from build123d import *

# Parameters (mm, degrees)
SKETCH1_R           = 10
SKETCH1_R_2         = 5
BOSS_EXTRUDE1_DEPTH = 3
SKETCH1_3_R         = 5
BOSS_EXTRUDE2_DEPTH = 27
CHAMFER1_SIZE       = 1
FILLET1_R           = 1


with BuildPart() as part:
    # Sketch1 → Boss-Extrude1 (new body)
    # profile 1 of 2: a face of its own
    with BuildSketch(Plane.XY):
        Circle(SKETCH1_R)
        Circle(SKETCH1_R_2, mode=Mode.SUBTRACT)
    # profile 2 of 2: a face of its own
    with BuildSketch(Plane.XY):
        Circle(SKETCH1_R_2)
    extrude(amount=BOSS_EXTRUDE1_DEPTH)

    # Sketch1_3 → Boss-Extrude2 (add)
    with BuildSketch(Plane.XY):
        Circle(SKETCH1_3_R)
    extrude(amount=BOSS_EXTRUDE2_DEPTH)

    # Chamfer1
    chamfer1_edges = [part.edges().sort_by_distance(p)[0] for p in [
        (-5, 0, 27),
    ]]
    chamfer(chamfer1_edges, length=CHAMFER1_SIZE)

    # Fillet1
    fillet1_edges = [part.edges().sort_by_distance(p)[0] for p in [
        (-10, 0, 0),
        (-10, 0, 3),
    ]]
    fillet(fillet1_edges, radius=FILLET1_R)


solid = part.part
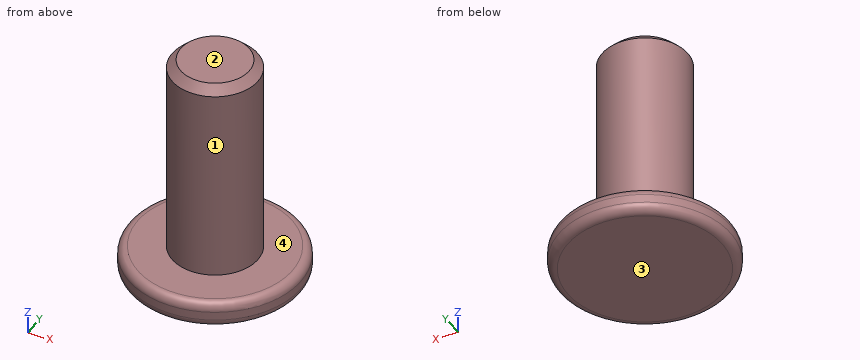
Verification items for the finished model (mm, model axes). Face numbers are marked on the shaded views. A direction names the side the tool comes from. Coordinates: 2 decimals unless noted, no trailing zeros. Order: outer loops, then holes, each group sorted by start corner. A loop starts at its lowest first (then second) coordinate and runs counter-clockwise, first axis right, second up. Notation, with made-up numbers: M -4.5,85 L 41.5,85 A20 ccw 41.5,108 Z; hole C -9.5,51 d1. An arc over 180 degrees is marked long. Write each question's results on one line, items separated by ' | '.
1) Access from +Z, -Z, +X, -X, +Y, -Y to the whole of each face (thin tool, end or side, straight path). Record for the marked faces 3 and 4.
Solved:
face 3: -Z, +X, -X, +Y, -Y | face 4: +Z
2) Scan lines: line 1 along Y through (x, z) = (3, 10); line 2 along Z through (x, y) = (-5, 3.75); line 3 along X through (y, z) = (2.5, 5.25). Record each from-to range of solid material in increasing order. Write a range as [from, to].
Solved:
line 1: y = [-4, 4] | line 2: z = [0, 3] | line 3: x = [-4.33, 4.33]
3) Gauge pin test, flat ends, axial feed: pin 1 Ø3 at (y, z) = (-5, 21.5) entering from -X; pin 2 Ø5.5 at (x, y) = (-4.5, -0.5) entering from +Z; pin 3 Ø5 at (y, z) = (-1, 19.5) entering from +X; pin 4 Ø6 at (x, z) = (6, 3) entering from -Y. Record the tip position at first contact, or that the pin passes through.
Solved:
pin 1: stops at x = -3.57 | pin 2: stops at z = 27 | pin 3: stops at x = 5 | pin 4: stops at y = -9.49
4) Section check C-C on z = 9.5. Record the cut outline in (x, y).
Solved:
outline: C 0,0 d10
5) Section check A-A on x = 0. Record the cut outline in (y, z), plus the area to 3 significant figures.
Solved:
outline: M -10,1 A1 ccw -9,0 L 9,0 A1 ccw 10,1 L 10,2 A1 ccw 9,3 L 5,3 L 5,26 L 4,27 L -4,27 L -5,26 L -5,3 L -9,3 A1 ccw -10,2 Z | area: 298 mm²
6) Release check for a two-part mould opening along X. For the marked faces 1 and 2 record: pulls with the +X half, pulls with the -X half, needs draft (parallel to the pull), parting line crosses it, or undercut.
Solved:
face 1: parting line crosses it | face 2: needs draft
